Part model, mm, in its own coordinate system. Round coordinates to 2 decimals unless told otherwise and drop trailing zeros. Order: outer loops, then holes, each group sorted by start corner. A loop starts at its lowest first (then second) coordinate and runs counter-clockwise, first axis right, second up. Notation, with made-up numbers: (-16.75, 77.25) -> (23.25, 77.25) arc R18 cw to (23.25, 84.25) -> close; hole circle Ø4 at (35.5, 22). An arc over 180 degrees is marked (long way). Answer as a JSON object with one key per item and string values. Group by question number.
Autodesk Fusion 360 part; units mm, degrees
sketch "Sketch1" plane through (0, 0, 0) normal (0, 0, 1) x (1, 0, 0)
  line L0 (0, 30) -> (72.9, 30)
  line L1 (72.9, 30) -> (72.9, -11.8)
  line L2 (72.9, -11.8) -> (0, -11.8)
  line L3 (0, -11.8) -> (0, 30)
  dimension "d1" = 72.9
  dimension "d2" = 41.8
extrude "Extrude1" add sketch "Sketch1" along normal blind 1
sketch "Sketch2" plane through (0, 0, 1) normal (0, 0, 1) x (-1, 0, 0)
  line L0 (0, 11.8) -> (-72.9, 11.8)
  line L1 (-72.9, 11.8) -> (-72.9, -30)
  line L2 (-72.9, -30) -> (0, -30)
  line L3 (0, -30) -> (0, 11.8)
  line L4 (0, -9.1) -> (-72.9, -9.1) construction
  line L5 (-72.9, -28.9) -> (-70.9, -28.9)
  line L6 (-70.9, -28.9) -> (-70.9, 10.7)
  line L7 (-70.9, 10.7) -> (-72.9, 10.7)
  line L8 (-72.9, 10.7) -> (-72.9, -28.9)
  dimension "d5" = 39.6
  dimension "d6" = 2
extrude "Extrude2" add sketch "Sketch2" along normal blind 1 contours L1 L5 L6 L7 L8
Q1. Band-saw the part on C-C (z = 1.3). List the corners of the cut face in (x, y), plus the area to 3 significant figures.
Q2. Drop flat-ended pins along their axis: pin 1 Ø0.8 at (x, z) = (72, 1.5) entering from +Y; pin 2 Ø21 at (x, y) = (34, 5.5) entering from +Z. Give the stop position or say it passes through.
Q3. Wall check: line 1 (Z direction, x = 28, y = 13); line 2 (X direction, y = 3.5, z = 1.25). Give the ranges that are in metal, low to high. Write a range as [from, to].
Q4. Band-saw the part on B-B (x = 8). List the corners of the cut face in (y, z), plus the area to 3 significant figures.
Q5. Band-saw the part on A-A (y = 27). List the corners of the cut face in (x, z), plus the area to 3 significant figures.
Completed:
{
 "1": {"outline": "(70.9, -10.7) -> (72.9, -10.7) -> (72.9, 28.9) -> (70.9, 28.9) -> close", "area": "79.2 mm2"},
 "2": {"pin 1": "y = 28.9", "pin 2": "z = 1"},
 "3": {"line 1": "[0, 1]", "line 2": "[70.9, 72.9]"},
 "4": {"outline": "(-11.8, 0) -> (30, 0) -> (30, 1) -> (-11.8, 1) -> close", "area": "41.8 mm2"},
 "5": {"outline": "(0, 0) -> (72.9, 0) -> (72.9, 2) -> (70.9, 2) -> (70.9, 1) -> (0, 1) -> close", "area": "74.9 mm2"}
}
